Read the model definition and answer for the solid it produces. Units are mm, in the model's axes. Face numbers are marked on the shaded views. A direction names the side the tool comes from. Give positions to 0.01 mm unless a question says otherwise; leave off trailing zeros. Order: outer loops, then holes, each group sorted by start corner. A loop starts at its lowest first (then second) coordinate and runs counter-clockwise, first axis right, second up.
```python
from build123d import *

# Parameters (mm, degrees)
BOSS_EXTRUDE2_DEPTH = 10
SKETCH2_W           = 250
SKETCH2_H           = 100
BOSS_EXTRUDE3_DEPTH = 4


with BuildPart() as part:
    # Sketch1 → Boss-Extrude2 (new body)
    with BuildSketch(Plane.XY):
        with BuildLine():
            Line((-49.595588235, 30.790441176), (-49.595588235, 55.790441176))
            Line((-49.595588235, 55.790441176), (-84.595588235, 55.790441176))
            Line((-84.595588235, 55.790441176), (-84.595588235, 5.790441176))
            Line((-84.595588235, 5.790441176), (-76.571127836, 5.790441176))
            Line((-76.571127836, 5.790441176), (-80.122995865, 8.369201143))
            Line((-80.122995865, 8.369201143), (-74.161024923, 10.431488509))
            ThreePointArc((-74.161024923, 10.431488509), (-65.548234046, 25.0391578), (-49.595588235, 30.790441176))
        make_face()
        with BuildLine():
            Line((10.404411765, 55.790441176), (-49.595588235, 55.790441176))
            Line((-49.595588235, 55.790441176), (-49.595588235, 30.790441176))
            ThreePointArc((-49.595588235, 30.790441176), (-46.420318597, 30.587974576), (-43.296479842, 29.983854194))
            Line((-43.296479842, 29.983854194), (-38.907655076, 38.5487403))
            Line((-38.907655076, 38.5487403), (-38.907655076, 28.390620042))
            ThreePointArc((-38.907655076, 28.390620042), (-30.648795615, 22.100531594), (-25.657089919, 12.997957973))
            Line((-25.657089919, 12.997957973), (-17.962154019, 12.997957973))
            Line((-17.962154019, 12.997957973), (-22.478851702, 5.790441176))
            Line((-22.478851702, 5.790441176), (-14.595588235, 5.790441176))
            ThreePointArc((-14.595588235, 5.790441176), (-12.499276658, 15.811471895), (-6.561903703, 24.151926396))
            Line((-6.561903703, 24.151926396), (-6.561903703, 35.084441479))
            Line((-6.561903703, 35.084441479), (0, 28.522537776))
            ThreePointArc((0, 28.522537776), (5.080053353, 30.216886016), (10.404411765, 30.790441176))
            Line((10.404411765, 30.790441176), (10.404411765, 55.790441176))
        make_face()
        with BuildLine():
            Line((70.404411765, 55.790441176), (10.404411765, 55.790441176))
            Line((10.404411765, 55.790441176), (10.404411765, 30.790441176))
            ThreePointArc((10.404411765, 30.790441176), (17.859813508, 29.652900917), (24.63674968, 26.343799964))
            Line((24.63674968, 26.343799964), (32.552494412, 30.790441176))
            Line((32.552494412, 30.790441176), (29.92126971, 21.41389329))
            ThreePointArc((29.92126971, 21.41389329), (33.993831518, 14.069286246), (35.404411765, 5.790441176))
            Line((35.404411765, 5.790441176), (45.404411765, 5.790441176))
            ThreePointArc((45.404411765, 5.790441176), (50.185133178, 20.493528384), (62.698873639, 29.573306483))
            Line((62.698873639, 29.573306483), (67.171172857, 38.5487403))
            Line((67.171172857, 38.5487403), (70.404411765, 30.790441176))
            Line((70.404411765, 30.790441176), (70.404411765, 55.790441176))
        make_face()
        with BuildLine():
            Line((130.404411765, 55.790441176), (70.404411765, 55.790441176))
            Line((70.404411765, 55.790441176), (70.404411765, 30.790441176))
            ThreePointArc((70.404411765, 30.790441176), (83.787720088, 26.906479118), (93.012607471, 16.461405843))
            Line((93.012607471, 16.461405843), (98.474145882, 18.660683713))
            Line((98.474145882, 18.660683713), (94.969848452, 10.431488509))
            ThreePointArc((94.969848452, 10.431488509), (95.295533849, 8.1211152), (95.404411765, 5.790441176))
            Line((95.404411765, 5.790441176), (105.404411765, 5.790441176))
            ThreePointArc((105.404411765, 5.790441176), (106.107781477, 11.678883811), (108.178312298, 17.23598627))
            Line((108.178312298, 17.23598627), (105.404411765, 23.549684511))
            Line((105.404411765, 23.549684511), (110.88755382, 21.41389329))
            ThreePointArc((110.88755382, 21.41389329), (119.578200582, 28.324707338), (130.404411765, 30.790441176))
            Line((130.404411765, 30.790441176), (130.404411765, 55.790441176))
        make_face()
        with BuildLine():
            Line((165.404411765, 55.790441176), (130.404411765, 55.790441176))
            Line((130.404411765, 55.790441176), (130.404411765, 30.790441176))
            ThreePointArc((130.404411765, 30.790441176), (133.401752606, 30.610109746), (136.355852267, 30.071717007))
            Line((136.355852267, 30.071717007), (140.818257218, 36.687543597))
            Line((140.818257218, 36.687543597), (142.579811014, 27.625267787))
            ThreePointArc((142.579811014, 27.625267787), (151.961139035, 18.451701358), (155.404411765, 5.790441176))
            Line((155.404411765, 5.790441176), (165.404411765, 5.790441176))
            Line((165.404411765, 5.790441176), (165.404411765, 55.790441176))
        make_face()
        with BuildLine():
            Line((165.404411765, -44.209558824), (165.404411765, 5.790441176))
            Line((165.404411765, 5.790441176), (155.404411765, 5.790441176))
            ThreePointArc((155.404411765, 5.790441176), (151.961139035, -6.870819005), (142.579811014, -16.044385434))
            Line((142.579811014, -16.044385434), (139.723435627, -21.807209952))
            Line((139.723435627, -21.807209952), (132.176529952, -19.14667167))
            ThreePointArc((132.176529952, -19.14667167), (131.291028602, -19.193832089), (130.404411765, -19.209558824))
            Line((130.404411765, -19.209558824), (130.404411765, -44.209558824))
            Line((130.404411765, -44.209558824), (165.404411765, -44.209558824))
        make_face()
        with BuildLine():
            ThreePointArc((78.603951233, -17.826661789), (74.562080934, -18.861410419), (70.404411765, -19.209558824))
            Line((70.404411765, -19.209558824), (70.404411765, -44.209558824))
            Line((70.404411765, -44.209558824), (130.404411765, -44.209558824))
            Line((130.404411765, -44.209558824), (130.404411765, -19.209558824))
            ThreePointArc((130.404411765, -19.209558824), (124.758153779, -18.563609221), (119.403671642, -16.659140484))
            Line((119.403671642, -16.659140484), (108.178312298, -21.807209952))
            Line((108.178312298, -21.807209952), (110.88755382, -9.833010937))
            ThreePointArc((110.88755382, -9.833010937), (106.814992011, -2.488403893), (105.404411765, 5.790441176))
            Line((105.404411765, 5.790441176), (95.404411765, 5.790441176))
            ThreePointArc((95.404411765, 5.790441176), (92.88136777, -5.154258396), (85.821495865, -13.889841287))
            Line((85.821495865, -13.889841287), (89.988841167, -19.209558824))
            Line((89.988841167, -19.209558824), (78.603951233, -17.826661789))
        make_face()
        with BuildLine():
            ThreePointArc((16.26584722, -18.512718585), (13.35576789, -19.034737514), (10.404411765, -19.209558824))
            Line((10.404411765, -19.209558824), (10.404411765, -44.209558824))
            Line((10.404411765, -44.209558824), (70.404411765, -44.209558824))
            Line((70.404411765, -44.209558824), (70.404411765, -19.209558824))
            ThreePointArc((70.404411765, -19.209558824), (66.503875434, -18.903400492), (62.698873639, -17.99242413))
            Line((62.698873639, -17.99242413), (57.774840306, -22.916457463))
            Line((57.774840306, -22.916457463), (57.774840306, -15.784867043))
            ThreePointArc((57.774840306, -15.784867043), (48.716404866, -6.644604331), (45.404411765, 5.790441176))
            Line((45.404411765, 5.790441176), (35.404411765, 5.790441176))
            ThreePointArc((35.404411765, 5.790441176), (32.092418663, -6.644604331), (23.033983223, -15.784867043))
            Line((23.033983223, -15.784867043), (24.63674968, -26.883621045))
            Line((24.63674968, -26.883621045), (16.26584722, -18.512718585))
        make_face()
        with BuildLine():
            ThreePointArc((-24.894580949, 1.935543121), (-33.337858557, -13.20129981), (-49.595588235, -19.209558824))
            Line((-49.595588235, -19.209558824), (-49.595588235, -44.209558824))
            Line((-49.595588235, -44.209558824), (10.404411765, -44.209558824))
            Line((10.404411765, -44.209558824), (10.404411765, -19.209558824))
            ThreePointArc((10.404411765, -19.209558824), (0.386918535, -17.114794674), (-7.951831841, -11.181545175))
            Line((-7.951831841, -11.181545175), (-15.042390882, -13.889841287))
            Line((-15.042390882, -13.889841287), (-11.571398063, -6.128610062))
            ThreePointArc((-11.571398063, -6.128610062), (-13.827749155, -0.357922603), (-14.595588235, 5.790441176))
            Line((-14.595588235, 5.790441176), (-22.478851702, 5.790441176))
            Line((-22.478851702, 5.790441176), (-24.894580949, 1.935543121))
        make_face()
        with BuildLine():
            Line((-76.571127836, 5.790441176), (-84.595588235, 5.790441176))
            Line((-84.595588235, 5.790441176), (-84.595588235, -44.209558824))
            Line((-84.595588235, -44.209558824), (-49.595588235, -44.209558824))
            Line((-49.595588235, -44.209558824), (-49.595588235, -19.209558824))
            ThreePointArc((-49.595588235, -19.209558824), (-55.612209406, -18.474765802), (-61.275152877, -16.313580398))
            Line((-61.275152877, -16.313580398), (-69.988075999, -18.512718585))
            Line((-69.988075999, -18.512718585), (-67.951831841, -11.181545175))
            ThreePointArc((-67.951831841, -11.181545175), (-72.598243173, -4.001283177), (-74.552596729, 4.324928615))
            Line((-74.552596729, 4.324928615), (-76.571127836, 5.790441176))
        make_face()
    extrude(amount=BOSS_EXTRUDE2_DEPTH)

    # Sketch2 → Boss-Extrude3 (add)
    with BuildSketch(Plane.XY.offset(10)):
        with Locations((40.404411765, 5.790441176)):
            Rectangle(SKETCH2_W, SKETCH2_H)
    extrude(amount=BOSS_EXTRUDE3_DEPTH)


solid = part.part
```
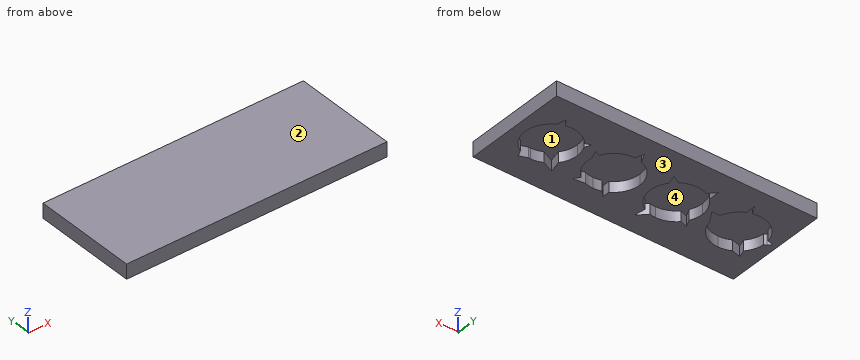
1) The part is cut by section A-A on z = 3.5. Count the separate pieces of the cut face and the enclosed holes in it, and give its area (3 significant figures).
Final values:
separate pieces: 1
enclosed holes: 4
area: 16,700 mm2
2) For a pull along Y with two mould halves and no side action, classify the marked faces 3 and 4 as released by +Y, released by -Y, zero draft, split by the parting line, or undercut.
Final values:
face 3: zero draft
face 4: undercut
3) Consider L1, parallel to Y at x = 131.5, z = 6.5; L2, parallel to X at y = 12, z = 3.5; L3, parallel to X at y = 27, z = 2.25. Determine where each line is inside the solid, lowest interval first.
Final values:
L1: y = -44.21 to -19.19, 30.77 to 55.79
L2: x = -84.6 to -73.81, -18.59 to -13.81, 34.62 to 46.19, 95.64 to 106.19, 154.62 to 165.4
L3: x = -84.6 to -62.83, -36.36 to -6.56, 23.64 to 25.8, 31.49 to 57.17, 83.64 to 117.17, 143.64 to 165.4
4) A tool of negligible diameter and unlimited length cuts with its end or side. For the marked faces 1 and 2, from which of +Z, -Z, +X, -X, +Y, -Y can it reach the whole face along a straight path? Write none if from no direction.
Final values:
face 1: -Z
face 2: +Z, +X, -X, +Y, -Y
5) The part is cut by section B-B on x = 150.5. Determine the outline of the cut face in (y, z).
Final values:
outline: (-44.21, 0) - (-9.08, 0) - (-9.08, 10) - (20.66, 10) - (20.66, 0) - (55.79, 0) - (55.79, 14) - (-44.21, 14) - close
6) Given pin 1 (4 mm diameter, centred on x = -11, y = -26.5, fed in from -Z); pin 2 (25 mm diameter, centred on x = 128, y = 9.5, fed in from -Z), each flat-ended and moving along its own axis, determine where each tip first touches the part or whether it passes through.
Final values:
pin 1: stops at z = 0
pin 2: stops at z = 10
